Design review of the part built by this model. Coordinates are the model's own, in mm. Face numbers are marked on the shaded views. A direction names the side the tool comes from. Coordinates: 2 decimals unless noted, no trailing zeros. Loops run counter-clockwise (first coordinate to the right, second up) from the corner with the lowest first, then second, coordinate; pieces in that order, holes last.
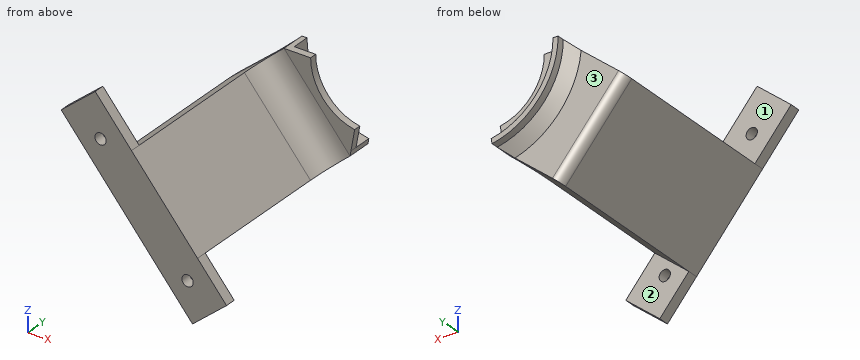
from build123d import *

# Parameters (mm, degrees)
BOSS_EXTRUDE1_DEPTH = 4
BOSS_EXTRUDE2_DEPTH = 14
BOSS_EXTRUDE3_DEPTH = 4
BOSS_EXTRUDE4_DEPTH = 103.5
FILLET1_R           = 15
FILLET2_R           = 5
CHAMFER1_SIZE       = 6
SKETCH6_W           = 25
SKETCH6_H           = 6
BOSS_EXTRUDE5_DEPTH = 25.4
SKETCH7_W           = 25
SKETCH7_H           = 6
BOSS_EXTRUDE6_DEPTH = 31.75
SKETCH8_R           = 2.5527
CUT_EXTRUDE1_DEPTH  = 25.4
SKETCH9_R           = 3.175
CUT_EXTRUDE2_DEPTH  = 25.4


with BuildPart() as part:
    # Sketch1 → Boss-Extrude1 (new body)
    with BuildSketch(Plane(origin=(0, 0, 0), x_dir=(1, 0, 0), z_dir=(0, 1, 0))):
        with BuildLine():
            Line((-42.1, 0), (-30, 0))
            ThreePointArc((-30, 0), (-22.981333, 19.283628), (-5.209445, 29.544233))
            Line((-5.209445, 29.544233), (-7.310588, 41.460406))
            ThreePointArc((-7.310588, 41.460406), (-32.250471, 27.061358), (-42.1, 0))
        make_face()
        with BuildLine():
            Line((-45, 0), (-42.1, 0))
            ThreePointArc((-42.1, 0), (-32.250471, 27.061358), (-7.310588, 41.460406))
            Line((-7.310588, 41.460406), (-7.814168, 44.316349))
            ThreePointArc((-7.814168, 44.316349), (-34.472, 28.925442), (-45, 0))
        make_face()
    extrude(amount=BOSS_EXTRUDE1_DEPTH)

    # Sketch1<3> → Boss-Extrude2 (add)
    with BuildSketch(Plane(origin=(0, 0, 0), x_dir=(1, 0, 0), z_dir=(0, 1, 0))):
        with BuildLine():
            Line((-45, 0), (-42.1, 0))
            ThreePointArc((-42.1, 0), (-32.250471, 27.061358), (-7.310588, 41.460406))
            Line((-7.310588, 41.460406), (-7.814168, 44.316349))
            ThreePointArc((-7.814168, 44.316349), (-34.472, 28.925442), (-45, 0))
        make_face()
    extrude(amount=BOSS_EXTRUDE2_DEPTH)

    # Sketch3 → Boss-Extrude3 (add)
    with BuildSketch(Plane.XZ):
        Polygon((-7.814168, -44.316349), (-45, 0), (-75.641778, -25.711504), (-38.455946, -70.027853), align=None)
    extrude(amount=-BOSS_EXTRUDE3_DEPTH)

    # Sketch4 → Boss-Extrude4 (add)
    with BuildSketch(Plane.XZ):
        Polygon((-38.455946, -70.027853), (-19.304835, -53.958163), (-56.490667, -9.641814), (-75.641778, -25.711504), align=None)
    extrude(amount=BOSS_EXTRUDE4_DEPTH)

    # Fillet1
    fillet1_edges = [part.edges().sort_by_distance(p)[0] for p in [
        (-37.897751, 0, -31.799989),
    ]]
    fillet(fillet1_edges, radius=FILLET1_R)

    # Fillet2
    fillet2_edges = [part.edges().sort_by_distance(p)[0] for p in [
        (-57.048862, 4, -47.869679),
    ]]
    fillet(fillet2_edges, radius=FILLET2_R)

    # Chamfer1
    chamfer1_edges = [part.edges().sort_by_distance(p)[0] for p in [
        (-34.472, 4, -28.925442),
    ]]
    chamfer(chamfer1_edges, length=CHAMFER1_SIZE)

    # Sketch6 → Boss-Extrude5 (add)
    with BuildSketch(Plane(origin=(18.592916, 0, -22.158174), x_dir=(-0.7660444431189766, 0, -0.6427876096865413), z_dir=(0.6427876096865411, 0, -0.7660444431189765))):
        with Locations((61.972, -100.5)):
            Rectangle(SKETCH6_W, SKETCH6_H)
    extrude(amount=BOSS_EXTRUDE5_DEPTH)

    # Sketch7 → Boss-Extrude6 (add)
    with BuildSketch(Plane(origin=(-18.592916, 0, 22.158174), x_dir=(0.7660444431189769, 0, 0.6427876096865406), z_dir=(-0.6427876096865406, 0, 0.7660444431189769))):
        with Locations((-61.972, -100.5)):
            Rectangle(SKETCH7_W, SKETCH7_H)
    extrude(amount=BOSS_EXTRUDE6_DEPTH)

    # Sketch8 → Cut-Extrude1 (cut)
    with BuildSketch(Plane(origin=(0, -97.5, 0), x_dir=(1, 0, 0), z_dir=(0, 1, 0))):
        with Locations(Location((-73.889481, 9.291988, 0), (0, 0, 270))):
            Circle(SKETCH8_R)
        with Locations(Location((-24.909065, 67.664575, 0), (0, 0, 270))):
            Circle(SKETCH8_R)
    extrude(amount=-CUT_EXTRUDE1_DEPTH, mode=Mode.SUBTRACT)

    # Sketch9 → Cut-Extrude2 (cut)
    with BuildSketch(Plane.XZ.offset(103.5)):
        with Locations(Location((-73.889481, -9.291988, 0), (0, 0, 270))):
            Circle(SKETCH9_R)
        with Locations(Location((-24.909065, -67.664575, 0), (0, 0, 270))):
            Circle(SKETCH9_R)
    extrude(amount=-CUT_EXTRUDE2_DEPTH, mode=Mode.SUBTRACT)


solid = part.part
Q1. For line 1 (Y direction, x = -62, z = -21); line 2 (Z direction, x = -53, y = -19); line 3 (X direction, y = -64.5, z = -19), list the stretches that pass through material, from the lowest coordinate up.
Q2. Machinability: for the marked faces 1, 2 and 3, which of the approach directions +Z, -Z, +X, -X, +Y, -Y give a long, thin tool a straight path to every point of the face, cutting with its end or side? Answer none if there is none.
Q3. Clearance check with flat-ended pins moving along their axes: pin 1 Ø5 at (x, y) = (-55.5, -85) entering from -Z; pin 2 Ø11 at (x, z) = (-27, -29) entering from +Y; pin 3 Ø8 at (y, z) = (-61, -40) entering from +X; pin 4 Ø8 at (y, z) = (-40, -69) entering from -X. State where each tip first meets the part, or that it passes through.
Q4. Take a section at B-B, the plane x = -87.5. Write out the cut boundary in (y, z), then the cut area to 3 significant figures.
Q5. Take a section at A-A, the plane y = -40.5. Write out the cut boundary in (x, z).
Entries:
1. line 1: y = -103.5 to 4
1. line 2: z = -52.69 to -13.8
1. line 3: x = -67.64 to -48.64
2. face 1: +Z, -X, +Y
2. face 2: -Z, +X, +Y
2. face 3: -Z, -X, +Y
3. pin 1: stops at z = -52.69
3. pin 2: stops at y = 14
3. pin 3: stops at x = -27.66
3. pin 4: stops at x = -42.67
4. outline: (-103.5, -11.58) - (-97.5, -11.58) - (-97.5, 5.78) - (-103.5, 5.78) - close
4. area: 104 mm2
5. outline: (-75.64, -25.71) - (-38.46, -70.03) - (-19.3, -53.96) - (-56.49, -9.64) - close
